```python
from build123d import *

# Parameters (mm, degrees)
F1_DEPTH = 5


with BuildPart() as f1:
    # F0 (on Top) → F1 (new body)
    with BuildSketch(Plane.XY):
        with BuildLine():
            Line((-4.25, 19.588463), (-4.25, -5.411537))
            ThreePointArc((-4.25, -5.411537), (0, -9.661537), (4.25, -5.411537))
            Line((4.25, -5.411537), (4.25, 19.588463))
            Line((4.25, 19.588463), (-4.25, 19.588463))
        make_face()
        with BuildLine():
            Line((-0.5, -1.947436), (-0.5, -2.962048))
            Line((-0.5, -2.962048), (-0.5, -7.861027))
            Line((-0.5, -7.861027), (-0.5, -8.875639))
            ThreePointArc((-0.5, -8.875639), (-3.5, -5.411537), (-0.5, -1.947436))
        make_face(mode=Mode.SUBTRACT)
        with BuildLine():
            Line((0.5, -7.861027), (0.5, -2.962048))
            Line((0.5, -2.962048), (0.5, -1.947436))
            ThreePointArc((0.5, -1.947436), (3.5, -5.411537), (0.5, -8.875639))
            Line((0.5, -8.875639), (0.5, -7.861027))
        make_face(mode=Mode.SUBTRACT)
    extrude(amount=F1_DEPTH)


solid = f1.part
```
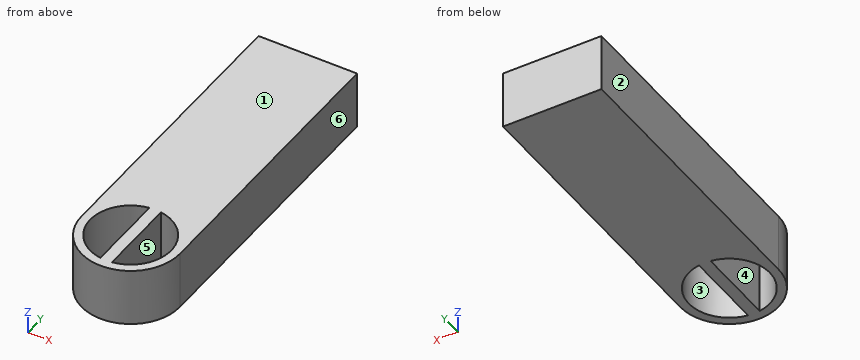
For this review, take the finished solid that the model builds, in its own axes (mm). Face numbers are marked on the shaded views. A direction names the side the tool comes from. Give positions to 0.01 mm unless a question says otherwise; leave off trailing zeros. Write each loop counter-clockwise with the first axis right and the second up, starting at its lowest first coordinate (ties: lowest second). Pieces come first, ordered by that corner, then holes. Notation, with made-up numbers: M -37,-7 L -13,-7 A19 cw -13,19 Z; hole C 64.25,19.25 d11. An arc over 180 degrees is marked long. One line per item, written item: value.
1) Take a section at C-C, the plane y = -6.5. Write out the cut boundary in (x, z).
Results are:
outline: M -4.11,0 L -3.33,0 L -3.33,5 L -4.11,5 Z; M -0.5,0 L 0.5,0 L 0.5,5 L -0.5,5 Z; M 3.33,0 L 4.11,0 L 4.11,5 L 3.33,5 Z
2) For P1, Ø1.5, axis at x = 2.5, y = 15.5, coming from the -Z side, flat-tipped, find the tip position at first contact; note if it passes through.
Results are:
P1: stops at z = 0
3) For line 1 (X direction, y = -3.5, z = 0.4); line 2 (X direction, y = -7.25, z = 1.6); line 3 (Y direction, x = 2.25, z = 0.6), list the stretches that pass through material, from the lowest coordinate up. Write a range as from..to.
Results are:
line 1: x = -4.25..-2.93, -0.5..0.5, 2.93..4.25
line 2: x = -3.83..-2.98, -0.5..0.5, 2.98..3.83
line 3: y = -9.02..-8.09, -2.73..19.59
4) Take a section at D-D, the plane x = -3. Write out the cut boundary in (y, z).
Results are:
outline: M -8.42,0 L -7.21,0 L -7.21,5 L -8.42,5 Z; M -3.61,0 L 19.59,0 L 19.59,5 L -3.61,5 Z
5) Take a section at A-A, the plane z = 2.95. Write out the cut boundary in (x, y).
Results are:
outline: M -4.25,-5.41 A4.25 ccw 4.25,-5.41 L 4.25,19.59 L -4.25,19.59 Z; hole M -0.5,-8.88 L -0.5,-1.95 A3.5 ccw Z; hole M 0.5,-8.88 A3.5 ccw 0.5,-1.95 Z
6) The part is to be moulded in two halves that separate along X. For the marked faces 1, 2, 3 and 4, say which applies: +X half, -X half, draft (parallel to the pull), parting line (faces both ways), or undercut.
Results are:
face 1: draft
face 2: -X half
face 3: undercut
face 4: undercut
7) Take a section at B-B, the plane x = 1.75. Write out the cut boundary in (y, z).
Results are:
outline: M -9.28,0 L -8.44,0 L -8.44,5 L -9.28,5 Z; M -2.38,0 L 19.59,0 L 19.59,5 L -2.38,5 Z
8) For the marked faces 5 and 6, list the 3-axis set-ups (+Z, -Z, +X, -X, +Y, -Y) from which the entire face can be reached by the end or side of a thin tool; tool diameter is ignored.
Results are:
face 5: +Z, -Z
face 6: +Z, -Z, +X, +Y, -Y
